```python
from build123d import *

# Parameters (mm, degrees)
F0_W     = 110.5
F0_H     = 50
F0_W_2   = 22
F0_H_2   = 30
F0_R     = 2
F0_W_3   = 27
F0_H_3   = 19
F1_DEPTH = 5
F2_W     = 110.5
F2_H     = 5
F3_DEPTH = 25
F4_R     = 2
F5_DEPTH = 5.001
F6_W     = 2
F6_H     = 30
F7_DEPTH = 50
F8_DEPTH = 5
F9_F1_R  = 2
F9_F2_R  = 1.9999


# Not quite as in the source:
# - a fillet or chamfer is up to 0.001 mm smaller than in the source, because OpenCascade refuses the exact size


with BuildPart() as f1:
    # F0 (on Top) → F1 (new body)
    with BuildSketch(Plane.XY):
        with Locations((34.25, 0)):
            Rectangle(F0_W, F0_H)
        Rectangle(F0_W_2, F0_H_2, mode=Mode.SUBTRACT)
        with Locations((39.5, 0)):
            Circle(F0_R, mode=Mode.SUBTRACT)
        with Locations((59.5, 0)):
            Rectangle(F0_W_3, F0_H_3, mode=Mode.SUBTRACT)
        with Locations((79.5, 0)):
            Circle(F0_R, mode=Mode.SUBTRACT)
    extrude(amount=F1_DEPTH)

    # F2 (on face) → F3 (join)
    with BuildSketch(Plane(origin=(0, 0, 0), x_dir=(1, 0, 0), z_dir=(0, 0, -1))):
        with Locations((34.25, -22.5)):
            Rectangle(F2_W, F2_H)
    extrude(amount=F3_DEPTH)

    # F4 (on face) → F5 (cut, through all)
    with BuildSketch(Plane.XZ.offset(-20)):
        with Locations((-16.5, -17)):
            Circle(F4_R)
        with Locations((-10.5, -17)):
            Circle(F4_R)
        with Locations((-4.5, -17)):
            Circle(F4_R)
    extrude(amount=-F5_DEPTH, mode=Mode.SUBTRACT)

    # F6 (on face) → F7 (join, through all)
    with BuildSketch(Plane(origin=(0, 25, 0), x_dir=(-1, 0, 0), z_dir=(0, 1, 0))):
        with Locations((22, -10)):
            Rectangle(F6_W, F6_H)
        with Locations((-90.5, -10)):
            Rectangle(F6_W, F6_H)
    extrude(amount=-F7_DEPTH)

    # F6 (on face) → F8 (join)
    with BuildSketch(Plane(origin=(0, 25, 0), x_dir=(-1, 0, 0), z_dir=(0, 1, 0))):
        with Locations((22, -10)):
            Rectangle(F6_W, F6_H)
        with Locations((-90.5, -10)):
            Rectangle(F6_W, F6_H)
    extrude(amount=F8_DEPTH)

    # F9: fillet of radius 2 on 10 edges, made by hand

    # F9_f1
    f9_f1_edges = [f1.edges().sort_by_distance(p)[0] for p in [
        (89.5, 20, -12.5),
        (34.25, 20, 0),
        (89.5, -2.5, 0),
        (-21, 20, -12.5),
        (-21, -2.5, 0),
    ]]
    fillet(f9_f1_edges, radius=F9_F1_R)

    # F9_f2 (radius 2 in the source; OpenCascade refuses exactly that, so slightly less here)
    f9_f2_edges = [f1.edges().sort_by_distance(p)[0] for p in [
        (34.25, -25, 0),
        (34.25, -25, 5),
        (89.5, -3.5, -25),
        (-23, 2.5, 5),
        (91.5, 2.5, 5),
        (88.9142135624, 19.4142135624, -25),
        (-20.4142135624, -25, -0.5857864376),
        (88.9142135624, -25, -0.5857864376),
    ]]
    fillet(f9_f2_edges, radius=F9_F2_R)


solid = f1.part
```
Geometry: final body of the model. Coordinates: model frame, mm. A direction names the side the tool comes from. Coordinates: 2 decimals unless noted, no trailing zeros. Order: outer loops, then holes, each group sorted by start corner. A loop starts at its lowest first (then second) coordinate and runs counter-clockwise, first axis right, second up. Notation, with made-up numbers: (14.5, 62) -> (42.5, 62) arc R14 ccw to (42.5, 87) -> close; hole circle Ø7 at (-27, 10). An arc over 180 degrees is marked (long way). Use CSV: the item, a comma, the result in double quotes.
1) Line query: line 1 (X direction, y = 25.5, z = -10.25); line 2 (Y direction, x = 79.5, z = 2); line 3 (Z direction, x = -10.5, y = 21.85). Output: solid intervals per line, ascending.
Findings:
line 1,"x = -23 to -21, 89.5 to 91.5"
line 2,"y = -25 to -2, 2 to 25"
line 3,"z = -24.99 to -19, -15 to 5"
2) Section A-A on x = 39.5. Output: boundary loops of the cut face in (y, z), then the cut area to 3 significant figures.
Findings:
outline,"(-25, 2) arc R2 ccw to (-23, 0) -> (-2, 0) -> (-2, 5) -> (-23, 5) arc R2 ccw to (-25, 3) -> close; (2, 0) -> (18, 0) arc R2 cw to (20, -2) -> (20, -23) arc R2 ccw to (22, -25) -> (25, -25) -> (25, 5) -> (2, 5) -> close"
area,"353 mm^2"
3) Section B-B on y = 0. State how many separate pieces and enclosed holes the cut face has, then the cut area to 3 significant figures.
Findings:
separate pieces,"5"
enclosed holes,"0"
area,"386 mm^2"
4) Pin query (flat end, axial travel): pin 1 Ø20.5 at (x, y) = (40, -7) entering from -Z; pin 2 Ø6 at (x, z) = (71, -12) entering from +Y. Return the tip coordinate at first contact, or that it passes through.
Findings:
pin 1,"stops at z = 0"
pin 2,"stops at y = 25"
5) Access query for faces 1 (the cylindrical face through (-16.76, 22.465, -15.017)), 2 (the cylindrical face through (-20.4, -2.21, -0.57)), 3 (the flat face through (89.5, 27, -10)), 4 (the flat face through (46, 0, 2)). Directions: +Z, -Z, +X, -X, +Y, -Y. A direction counts if a zero-diameter tool reaches every point of the face in a straight line with its end or side. Return the directions, or none.
Findings:
face 1,"+Y, -Y"
face 2,"-Z, -Y"
face 3,"+Z, -Z, +Y"
face 4,"+Z, -Z"
6) Mould query, pull axis X, two halves, no side actions, for faces 5 (the flat face through (35, -3, 5)), 6 (the cylindrical face through (90.9, 2.89, 4.43)), 7 (the cylindrical face through (-21.6, -24.43, -13.34)). Classes: +X half, -X half, draft (parallel to the pull), parting line (faces both ways), or undercut.
Findings:
face 5,"draft"
face 6,"+X half"
face 7,"undercut"
